Autodesk Inventor part; units mm, degrees
ref_plane "YZ Plane" through (0, 0, 0) normal (1, 0, 0) x (0, 1, 0)
ref_plane "XZ Plane" through (0, 0, 0) normal (0, 1, 0) x (-1, 0, 0)
ref_plane "XY Plane" through (0, 0, 0) normal (0, 0, 1) x (1, 0, 0)
sketch "Sketch1" plane through (0, 0, 0) normal (0, 1, 0) x (-1, 0, 0)
  line L0 (305.435, 114.3) -> (-305.435, 114.3)
  line L1 (-305.435, 114.3) -> (-305.435, -114.3)
  line L2 (-305.435, -114.3) -> (305.435, -114.3)
  line L3 (305.435, -114.3) -> (305.435, 114.3)
  line L4 (305.435, 114.3) -> (-305.435, -114.3) construction
  line L5 (-305.435, 114.3) -> (305.435, -114.3) construction
  point P0 (0, 0)
  dimension "d0" = 610.87
  dimension "d1" = 228.6
extrude "Extrusion1" add sketch "Sketch1" along normal mid plane 1.5875
sketch "Sketch2" plane through (0, 0.7937, 0) normal (0, 1, 0) x (1, 0, 0)
  circle A0 centre (200, 0) radius 16
  circle A1 centre (264, -64) radius 2.5 construction
  circle A2 centre (270, -70) radius 2
  circle A3 centre (270, -58) radius 2
  circle A4 centre (258, -58) radius 2
  circle A5 centre (258, -70) radius 2
  circle A6 centre (258, 58) radius 2
  circle A7 centre (270, 58) radius 2
  circle A8 centre (270, 70) radius 2
  circle A9 centre (258, 70) radius 2
  circle A10 centre (142, 58) radius 2
  circle A11 centre (142, 70) radius 2
  circle A12 centre (130, 70) radius 2
  circle A13 centre (130, 58) radius 2
  circle A14 centre (142, -58) radius 2
  circle A15 centre (130, -58) radius 2
  circle A16 centre (130, -70) radius 2
  circle A17 centre (142, -70) radius 2
  point P0 (0, 0)
  dimension "d4" = 32
  dimension "d5" = 200
  dimension "d6" = 5
  dimension "d7" = 64
  dimension "d8" = 64
  dimension "d11" = 4
  dimension "d12" = 6
  dimension "d13" = 6
  dimension "d16" = 360
  dimension "d20" = 360
extrude "Extrusion2" cut sketch "Sketch2" against normal through all
sketch "Sketch3" plane through (0, 0.7937, 0) normal (0, 1, 0) x (1, 0, 0)
  circle A0 centre (-56, 0) radius 7 construction
  circle A1 centre (200, 0) radius 16 construction
  circle A2 centre (-96, -40) radius 2.5 construction
  circle A3 centre (-90, -34) radius 2
  circle A4 centre (-102, -34) radius 2
  circle A5 centre (-102, -46) radius 2
  circle A6 centre (-90, -46) radius 2
  circle A7 centre (-22, -46) radius 2
  circle A8 centre (-22, -34) radius 2
  circle A9 centre (-10, -46) radius 2
  circle A10 centre (-10, -34) radius 2
  circle A11 centre (-10, 34) radius 2
  circle A12 centre (-22, 34) radius 2
  circle A13 centre (-10, 46) radius 2
  circle A14 centre (-22, 46) radius 2
  circle A15 centre (-90, 46) radius 2
  circle A16 centre (-90, 34) radius 2
  circle A17 centre (-102, 46) radius 2
  circle A18 centre (-102, 34) radius 2
  point P0 (0, 0)
  dimension "d24" = 14
  dimension "d25" = 256
  dimension "d42" = 5
  dimension "d43" = 40
  dimension "d44" = 40
  dimension "d45" = 4
  dimension "d46" = 6
  dimension "d47" = 6
  dimension "d50" = 360
  dimension "d54" = 360
extrude "Extrusion4" cut sketch "Sketch3" against normal through all
properties part number "ChassisTop"
Could you check a few things on this model? Use its own coordinates, in mm. Give positions to 0.01 mm unless a question says otherwise; leave off trailing zeros. Return JSON: item names as keys, results as strings.
1. Thinking about a two-plate mould opening in Z: for faces 1 (the flat face through (4, 0.794, 2)), 2 (the cylindrical face through (184.015, 0.011, -0.703)), which applies, pulls with the +Z half, pulls with the -Z half, needs draft (parallel to the pull), parting line crosses it, or undercut?
Answer list:
{"face 1": "needs draft", "face 2": "undercut"}
2. I need wall thicknesses on line 1 (X direction, y = 0.4, z = 46) (3 decimals); line 2 (Z direction, x = 130, y = -0.2); line 3 (X direction, y = 0.35, z = 58) (3 decimals). Which ranges of each line are inside material? Lowest first, please. Write a range as from..to.
Answer list:
{"line 1": "x = -305.435..-104, -100..-92, -88..-24, -20..-12, -8..305.435", "line 2": "z = -114.3..-72, -68..-60, -56..56, 60..68, 72..114.3", "line 3": "x = -305.435..128, 132..140, 144..256, 260..268, 272..305.435"}
3. For pin 1 Ø3 at (x, z) = (-10, -34) entering from +Y, with a flat end and sliding along its axis, tell me the tip position at first contact or that it passes through.
Answer list:
{"pin 1": "passes through"}
